Read the model definition and answer for the solid it produces. Units are mm, in the model's axes. Coordinates: 2 decimals unless noted, no trailing zeros. Write each loop counter-clockwise with the first axis right and the second up, starting at its lowest first coordinate (ties: lowest second). Pieces come first, ordered by that corner, then holes.
(1) Given pin 1 (5 mm diameter, centred on x = 18.5, z = -6, fed in from -Y); pin 2 (0.8 mm diameter, centred on y = -2.5, z = -11.5, fed in from +X); pin 3 (1.8 mm diameter, centred on y = -2.5, z = -11, fed in from -X), each flat-ended and moving along its own axis, determine where each tip first touches the part or whether it passes through.
(2) Straight lines are drawn through the part: line 1 along X through (y, z) = (-1.75, -5.5); line 2 along Y through (x, z) = (22.75, -15.75); line 3 along X through (y, z) = (-5.5, -16.25). For each, find the intervals that lie inside material, in ascending order.
(3) The part is cut by section B-B, the plane y = -4.5. Determine the outline of the cut face in (x, z), and give its area (3 significant figures).
(4) The part is cut by section A-A, the plane y = -2. Determine the outline of the cut face in (x, z), and give its area (3 significant figures).
```python
from build123d import *

# Parameters (mm, degrees)
BOSS_EXTRUDE1_DEPTH = 18


with BuildPart() as part:
    # Sketch1 → Boss-Extrude1 (new body)
    with BuildSketch(Plane.XY):
        with BuildLine():
            Line((35.376892046, -6.781044394), (36.866346672, -6.277070186))
            Line((36.866346672, -6.277070186), (36.834295551, -6.182345714))
            Line((36.834295551, -6.182345714), (35.085481214, -3.589621837))
            ThreePointArc((35.085481214, -3.589621837), (35.021847622, -3.456211238), (35, -3.310025385))
            Line((35, -3.310025385), (35, -1.682345714))
            ThreePointArc((35, -1.682345714), (34.853553391, -1.328792323), (34.5, -1.182345714))
            Line((34.5, -1.182345714), (11.5, -1.182345714))
            ThreePointArc((11.5, -1.182345714), (11.146446609, -1.328792323), (11, -1.682345714))
            Line((11, -1.682345714), (11, -3.310025385))
            ThreePointArc((11, -3.310025385), (10.978152378, -3.456211238), (10.914518786, -3.589621837))
            Line((10.914518786, -3.589621837), (9.165704449, -6.182345714))
            Line((9.165704449, -6.182345714), (9.133653328, -6.277070186))
            Line((9.133653328, -6.277070186), (10.607058659, -6.77561393))
            add(Edge.make_bspline(
                [(10.607058659, -6.77561393), (11.816063951, -7.18469486), (13.628034684, -7.692085525), (16.113891162, -8.202802822), (18.189551086, -8.532681309), (20.512287403, -8.80284347), (22.525873147, -8.895511296), (24.157727683, -8.851859587), (25.351258415, -8.774619539), (26.610405964, -8.65564999), (28.052887591, -8.489315058), (29.715436425, -8.277918045), (32.229421821, -7.855388776), (34.119164741, -7.321218718), (35.376892046, -6.781044394)],
                knots=[0, 0, 0, 0, 0.14631509, 0.222398937, 0.304823105, 0.398352424, 0.499675853, 0.544569926, 0.593205172, 0.641840418, 0.694528601, 0.764759844, 0.840843691, 1, 1, 1, 1], degree=3, weights=[1, 1, 1, 1, 1, 1, 1, 1, 1, 1, 1, 1, 1, 1, 1]))
        make_face()
    extrude(amount=-BOSS_EXTRUDE1_DEPTH)


solid = part.part
```
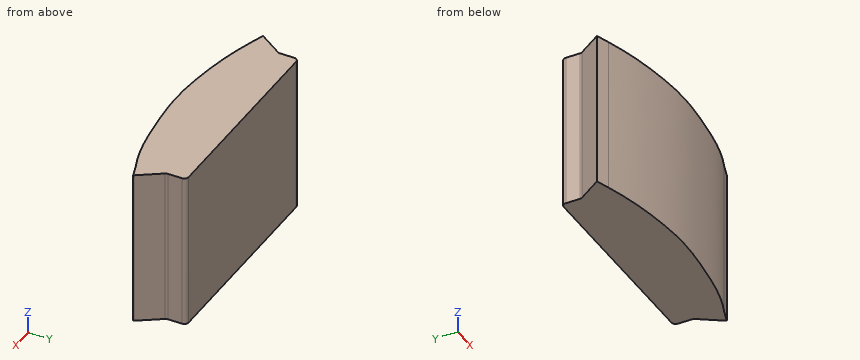
Computed:
1. pin 1: stops at y = -8.81
1. pin 2: stops at x = 35
1. pin 3: stops at x = 10.99
2. line 1: x = 11 to 35
2. line 2: y = -8.87 to -1.18
2. line 3: x = 9.63 to 36.37
3. outline: (10.3, -18) - (35.7, -18) - (35.7, 0) - (10.3, 0) - close
3. area: 457 mm2
4. outline: (11, -18) - (35, -18) - (35, 0) - (11, 0) - close
4. area: 432 mm2
